from build123d import *

# Parameters (mm, degrees)
ESBO_O2_R                  = 17.5
RESSALTO_EXTRUS_O2_DEPTH   = 8
CORTE_EXTRUS_O2_DEPTH      = 27.009613607
CORTE_EXTRUS_O2_DEPTH_BACK = 27.009613607
ESBO_O6_R                  = 2
ESBO_O7_R                  = 9
ESBO_O7_R_2                = 6
RESSALTO_EXTRUS_O3_DEPTH   = 14
CORTE_EXTRUS_O3_DEPTH      = 29.434134416
CORTE_EXTRUS_O3_DEPTH_BACK = 29.434134416
ESBO_O8_R                  = 6


with BuildPart() as part:
    # Esboço2 → Ressalto-extrusão2 (new body)
    with BuildSketch(Plane.XY):
        Circle(ESBO_O2_R)
    extrude(amount=RESSALTO_EXTRUS_O2_DEPTH)

    # Esboço6 → Corte-extrusão2 (cut, two sides: drawn at the far end of the back side and taken through both)
    with BuildSketch(Plane.XY.offset(8).offset(-CORTE_EXTRUS_O2_DEPTH_BACK)):
        with Locations((0, 14.523179991)):
            Circle(ESBO_O6_R)
        with Locations((14.523179991, 0)):
            Circle(ESBO_O6_R)
        with Locations((0, -14.523179991)):
            Circle(ESBO_O6_R)
        with Locations((-14.523179991, 0)):
            Circle(ESBO_O6_R)
    extrude(amount=CORTE_EXTRUS_O2_DEPTH + CORTE_EXTRUS_O2_DEPTH_BACK, mode=Mode.SUBTRACT)

    # Esboço7 → Ressalto-extrusão3 (add)
    with BuildSketch(Plane.XY.offset(8)):
        Circle(ESBO_O7_R)
        Circle(ESBO_O7_R_2, mode=Mode.SUBTRACT)
    extrude(amount=RESSALTO_EXTRUS_O3_DEPTH)

    # Esboço8 → Corte-extrusão3 (cut, two sides: drawn at the far end of the back side and taken through both)
    with BuildSketch(Plane.XY.offset(8).offset(-CORTE_EXTRUS_O3_DEPTH_BACK)):
        Circle(ESBO_O8_R)
    extrude(amount=CORTE_EXTRUS_O3_DEPTH + CORTE_EXTRUS_O3_DEPTH_BACK, mode=Mode.SUBTRACT)


solid = part.part
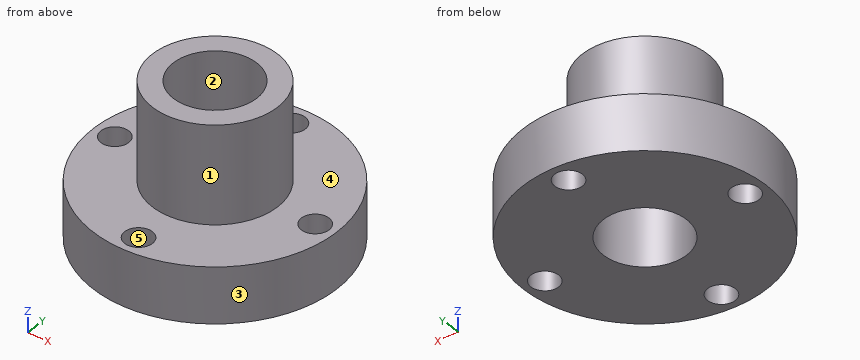
Model file for the job. Use its own axes, mm. Face numbers are marked on the shaded views. A direction names the side the tool comes from. Round coordinates to 2 decimals unless told otherwise and drop trailing zeros. Order: outer loops, then holes, each group sorted by start corner. A loop starts at its lowest first (then second) coordinate and runs counter-clockwise, first axis right, second up.
(1) Band-saw the part on C-C (y = -15). List the corners of the cut face in (x, z), then the cut area to 3 significant figures.
(2) Band-saw the part on A-A (y = 0). List the corners of the cut face in (x, z).
(3) Pin check, flat tips, straight feed: pin 1 (12 mm diameter, centred on x = -9, z = 8, fed in from +Y); pin 2 (4 mm diameter, centred on x = 12, z = 19.5, fed in from -Y); pin 3 (3 mm diameter, centred on x = -4, z = 18.5, fed in from +Y); pin 4 (4.5 mm diameter, centred on x = -14.52, y = 0, fed in from +Z). Stop position of each tip, or through.
(4) Band-saw the part on D-D (z = 19). List the corners of the cut face in (x, y).
(5) Drill centre lines: line 1 (Y direction, x = 0, z = 4.5); line 2 (X direction, y = -1.5, z = 7.5); line 3 (Y direction, x = -1, z = 6). Where is each one in solid material? Low to high.
(6) 3-axis set-ups, long thin cutter, end or side, ignore diameter. For the marked faces 1 and 2: which of +Z, -Z, +X, -X, +Y, -Y reach the whole face in a straight line?
(7) Pull direction Y, two halves, no side cores. Call the marked faces 3, 4 and 5: released by +Y, released by -Y, zero draft, split by the parting line, or undercut.
Verdict:
1. outline: (-9.01, 0) - (-1.94, 0) - (-1.94, 8) - (-9.01, 8) - close; (1.94, 0) - (9.01, 0) - (9.01, 8) - (1.94, 8) - close
1. area: 113 mm2
2. outline: (-17.5, 0) - (-16.52, 0) - (-16.52, 8) - (-17.5, 8) - close; (-12.52, 0) - (-6, 0) - (-6, 22) - (-9, 22) - (-9, 8) - (-12.52, 8) - close; (6, 0) - (12.52, 0) - (12.52, 8) - (9, 8) - (9, 22) - (6, 22) - close; (16.52, 0) - (17.5, 0) - (17.5, 8) - (16.52, 8) - close
3. pin 1: stops at y = 17.24
3. pin 2: passes through
3. pin 3: stops at y = 8.65
3. pin 4: stops at z = 8
4. outline: circle Ø18 at (0, 0); hole circle Ø12 at (0, 0)
5. line 1: y = -17.5 to -16.52, -12.52 to -6, 6 to 12.52, 16.52 to 17.5
5. line 2: x = -17.44 to -15.85, -13.2 to -5.81, 5.81 to 13.2, 15.85 to 17.44
5. line 3: y = -17.47 to -16.26, -12.79 to -5.92, 5.92 to 12.79, 16.26 to 17.47
6. face 1: +Z
6. face 2: +Z, -Z
7. face 3: split by the parting line
7. face 4: zero draft
7. face 5: undercut
